Source: three-view drawing plus pictorial views. Frame: mm from the lowest corner of the part. Give positions to 0.01 mm unless a question says otherwise; leave off trailing zeros. Loops run counter-clockwise (first coordinate to the right, second up) from the corner with the lowest first, then second, coordinate; pieces in that order, holes last. Notation, with made-up numbers: M 66.5,73.25 L 86.5,73.25 A19 ccw 86.5,95.25 Z; hole C 46,-8.5 d2. An arc over 180 degrees is marked long. One line per item, written item: value. Start each with the question number.
(1) Ray query, line 1 along Z through (x, y) = (13, 4.25); line 2 along Z through (x, y) = (4.5, 4.75); line 3 along X through (y, z) = (3, 23). Return the intervals inside material, ascending. Write a range as from..to.
(2) Section B-B on y = 5.5. Output: boundary loops of the cut face in (x, z).
(3) Section D-D on x = 2.25. Output: boundary loops of the cut face in (y, z).
(4) Section C-C on z = 63. Output: boundary loops of the cut face in (x, y).
(5) Section A-A on x = 13. Output: boundary loops of the cut face in (y, z), plus the area to 3 significant figures.
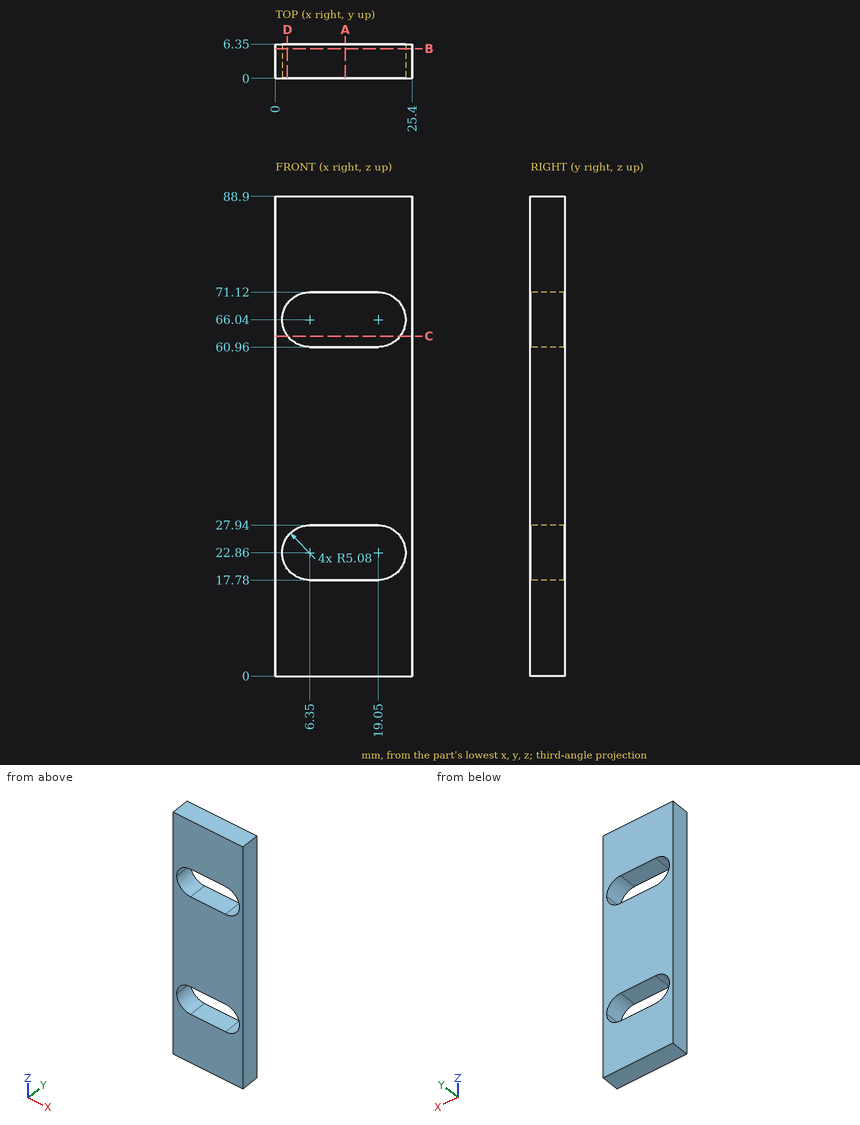
Output values:
1. line 1: z = 0..17.78, 27.94..60.96, 71.12..88.9
1. line 2: z = 0..18.13, 27.59..61.31, 70.77..88.9
1. line 3: x = 0..1.27, 24.13..25.4
2. outline: M 0,0 L 25.4,0 L 25.4,88.9 L 0,88.9 Z; hole M 6.35,17.78 L 19.05,17.78 A5.08 ccw 19.05,27.94 L 6.35,27.94 A5.08 ccw Z; hole M 6.35,60.96 L 19.05,60.96 A5.08 ccw 19.05,71.12 L 6.35,71.12 A5.08 ccw Z
3. outline: M 0,0 L 6.35,0 L 6.35,19.86 L 0,19.86 Z; M 0,25.86 L 6.35,25.86 L 6.35,63.04 L 0,63.04 Z; M 0,69.04 L 6.35,69.04 L 6.35,88.9 L 0,88.9 Z
4. outline: M 0,0 L 2.28,0 L 2.28,6.35 L 0,6.35 Z; M 23.12,0 L 25.4,0 L 25.4,6.35 L 23.12,6.35 Z
5. outline: M 0,0 L 6.35,0 L 6.35,17.78 L 0,17.78 Z; M 0,27.94 L 6.35,27.94 L 6.35,60.96 L 0,60.96 Z; M 0,71.12 L 6.35,71.12 L 6.35,88.9 L 0,88.9 Z
5. area: 435 mm²
